Can you work these out from the model? Positions are in its coordinate system, mm. Face numbers are marked on the shaded views. A direction names the side the tool comes from. Give positions to 0.01 mm unless a question says otherwise; leave off trailing zeros. Loops run counter-clockwise (first coordinate to the right, second up) from the corner with the lowest first, then second, coordinate; pieces in that order, holes last. Notation, with made-up numbers: M 21.25,53.5 L 78.25,53.5 A14 ccw 78.25,64.5 Z; hole C 13,27 d8. An arc over 180 degrees is marked long. One line per item, written item: value. Start each with the question number.
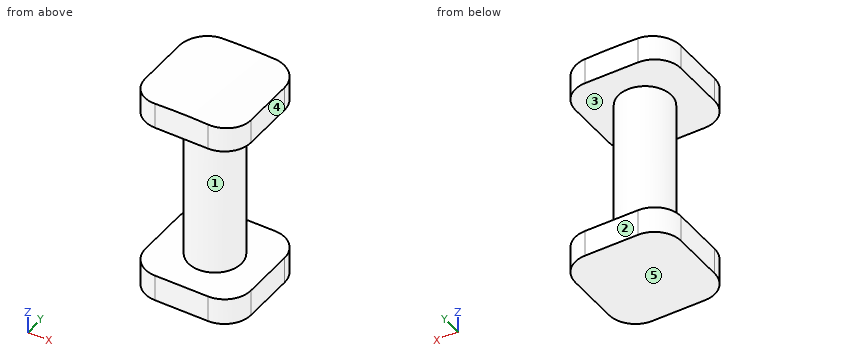
from build123d import *

# Parameters (mm, degrees)
F1_DEPTH = 25.4
F4_DEPTH = 25.4
F5_R     = 50.8
F6_DEPTH = 25.4
F7_W     = 11.8262093864
F7_H     = 19.0586867377


with BuildPart() as f1:
    # F0 (on Top) → F1 (new body)
    with BuildSketch(Plane.XY):
        with BuildLine():
            ThreePointArc((6.35, 3.175), (5.4200640303, 5.4200640303), (3.175, 6.35))
            Line((3.175, 6.35), (-3.175, 6.35))
            ThreePointArc((-3.175, 6.35), (-5.4200640303, 5.4200640303), (-6.35, 3.175))
            Line((-6.35, 3.175), (-6.35, -3.175))
            ThreePointArc((-6.35, -3.175), (-5.4200640303, -5.4200640303), (-3.175, -6.35))
            Line((-3.175, -6.35), (3.175, -6.35))
            ThreePointArc((3.175, -6.35), (5.4200640303, -5.4200640303), (6.35, -3.175))
            Line((6.35, -3.175), (6.35, 3.175))
        make_face()
    extrude(amount=F1_DEPTH)

    # F3 (on offset) → F4 (cut)
    with BuildSketch(Plane.XZ.offset(6.35)):
        with BuildLine():
            ThreePointArc((-43.2637086009, 11.9271194787), (1.858689826, 25.3773278091), (46.2714276243, 9.7425056106))
            Line((46.2714276243, 9.7425056106), (46.1867414415, 53.5595417023))
            Line((46.1867414415, 53.5595417023), (-43.2637086009, 53.5595417023))
            Line((-43.2637086009, 53.5595417023), (-43.2637086009, 11.9271194787))
        make_face()
    extrude(amount=-F4_DEPTH, mode=Mode.SUBTRACT)

    # F5 (on offset) → F6 (cut)
    with BuildSketch(Plane.XZ.offset(6.35)):
        with Locations((0, -50.8)):
            Circle(F5_R)
    extrude(amount=-F6_DEPTH, mode=Mode.SUBTRACT)

    # F7 (on Front) → F8 (revolve, cut)
    with BuildSketch(Plane.XZ):
        with Locations((9.0881046932, 12.7043433689)):
            Rectangle(F7_W, F7_H)
    revolve(axis=Axis((0, 0, 19.7457969189), (0, 0, -1)), mode=Mode.SUBTRACT)


solid = f1.part
Q1. If we section it at C-C, the plane y = 0: Write out the boundary of the cut face in (x, z) (3 decimals), plus the area to 3 significant figures.
Q2. Which directions (+Z, -Z, +X, -X, +Y, -Y) give clear straight access to the entire face, cutting with the end or side of a thin tool? Please do the marked faces 1 and 2.
Q3. If we section it at B-B, the plane y = 4.25: Write out the boundary of the cut face in (x, z) (3 decimals), plus the area to 3 significant figures.
Q4. For P1, Ø2, axis at x = 0, z = 6, coming from the -Y side (3 decimals); P2, Ø1.5, axis at y = 2, z = 14, coming from the +X side; P3, Ø6, axis at x = -1.5, z = 14.5, coming from the +Y side (3 decimals), each with a flat end and sliding along its axis, tell me the tip position at first contact or that it passes through.
Q5. If we mould it in two halves opening along Z, with no side actions, what happens to the marked faces 3, 4 and 5? For each: released by +Z, released by -Z, zero draft, split by the parting line, or undercut.
Q6. If we section it at A-A, the plane x = 4: Write out the boundary of the cut face in (y, z) (3 decimals).
Q7. If we section it at D-D, the plane x = 0: Write out the boundary of the cut face in (y, z) (3 decimals), plus the area to 3 significant figures.
Q8. I need wall thicknesses on line 1 along Z through (x, y) = (-3.25, -1.5) (3 decimals); line 2 along Z through (x, y) = (3, 0.5); line 3 along Z through (x, y) = (0.5, 4.25) (3 decimals). Which ranges of each line are inside material? Lowest first, please.
Response:
1. outline: M -6.35,0 L 6.35,0 L 6.35,3.175 L 3.175,3.175 L 3.175,22.234 L 6.35,22.234 L 6.35,25.135 A76.2 ccw -6.35,25.135 L -6.35,22.234 L -3.175,22.234 L -3.175,3.175 L -6.35,3.175 Z
1. area: 200 mm^2
2. face 1: none
2. face 2: +Z, -Z, +X, -X, +Y
3. outline: M -6.162,0 L 6.162,0 L 6.162,3.175 L -6.162,3.175 Z; M -6.162,22.234 L 6.162,22.234 L 6.162,25.15 A76.2 ccw -6.162,25.15 Z
3. area: 77.1 mm^2
4. P1: y = -3.175
4. P2: x = 2.92
4. P3: y = 3.175
5. face 3: undercut
5. face 4: zero draft
5. face 5: released by -Z
6. outline: M -6.241,0 L 6.241,0 L 6.241,3.175 L -6.241,3.175 Z; M -6.241,22.234 L 6.241,22.234 L 6.241,25.295 L -6.241,25.295 Z
7. outline: M -6.35,0 L 6.35,0 L 6.35,3.175 L 3.175,3.175 L 3.175,22.234 L 6.35,22.234 L 6.35,25.4 L -6.35,25.4 L -6.35,22.234 L -3.175,22.234 L -3.175,3.175 L -6.35,3.175 Z
7. area: 202 mm^2
8. line 1: 0 to 3.175, 22.234 to 25.331
8. line 2: 0 to 25.34
8. line 3: 0 to 3.175, 22.234 to 25.398
